Can you work these out from the model? Positions are in its coordinate system, mm. A direction names the side the tool comes from. Round coordinates to 2 decimals unless told otherwise and drop trailing zeros. Order: outer loops, then holes, each group sorted by start corner. A loop starts at its lowest first (then second) coordinate and runs counter-clockwise, first axis right, second up. Notation, with made-up numbers: (24, 29) - (75, 29) arc R22 cw to (75, 46) - close; hole circle Ø3 at (59.5, -22). An arc over 180 degrees is marked (long way). Write item = value, one per line.
from build123d import *

# Parameters (mm, degrees)
SKETCH1_R            = 3.5
BOSS_EXTRUDE1_DEPTH  = 5
SKETCH12_R           = 8.25
SKETCH12_R_2         = 3.5
BOSS_EXTRUDE6_DEPTH  = 5
BOSS_EXTRUDE9_DEPTH  = 5
CIRPATTERN2_COUNT    = 10
CUT_EXTRUDE1_START   = -10
SKETCH14_R           = 3.5
CUT_EXTRUDE1_DEPTH   = 10
SKETCH17_R           = 8.25
SKETCH17_R_2         = 3.5
BOSS_EXTRUDE10_DEPTH = 18


with BuildPart() as part:
    # Sketch1 → Boss-Extrude1 (new body)
    with BuildSketch(Plane(origin=(0, 0, 0), x_dir=(1, 0, 0), z_dir=(0, 1, 0))):
        with Locations(Location((0, 0, 0), (0, 0, 270))):
            Circle(SKETCH1_R)
    extrude(amount=BOSS_EXTRUDE1_DEPTH)

    # Sketch14 → Cut-Extrude1 (cut)
    with BuildSketch(Plane(origin=(0, 5, 0), x_dir=(1, 0, 0), z_dir=(0, 1, 0)).offset(CUT_EXTRUDE1_START)):
        with Locations(Location((0, 0, 0), (0, 0, 90))):
            Circle(SKETCH14_R)
    extrude(amount=CUT_EXTRUDE1_DEPTH, mode=Mode.SUBTRACT)


with BuildPart() as body_2:
    # Sketch12 → Boss-Extrude6 (new body)
    with BuildSketch(Plane(origin=(0, 5, 0), x_dir=(-1, 0, 0), z_dir=(0, -1, 0))):
        with Locations(Location((0, 0, 0), (0, 0, 90))):
            Circle(SKETCH12_R)
        with Locations(Location((0, 0, 0), (0, 0, 90))):
            Circle(SKETCH12_R_2, mode=Mode.SUBTRACT)
    extrude(amount=BOSS_EXTRUDE6_DEPTH)



with BuildPart() as body_3:
    # Sketch13 → Boss-Extrude9 (new body)
    with BuildSketch(Plane.XZ):
        with BuildLine():
            Line((1.7, 8.072948656), (0.86, 10.213858233))
            Line((0.86, 10.213858233), (-0.86, 10.213858233))
            Line((-0.86, 10.213858233), (-1.7, 8.072948656))
            ThreePointArc((-1.7, 8.072948656), (0, 8.25), (1.7, 8.072948656))
        make_face()
    extrude(amount=-BOSS_EXTRUDE9_DEPTH)


with BuildPart() as cirpattern2_1:
    # CirPattern2: pattern copy
    add(body_3.part.rotate(Axis((0, 0, 0), (0, 1, 0)), 1 * 360 / CIRPATTERN2_COUNT))


with BuildPart() as cirpattern2_2:
    # CirPattern2: pattern copy
    add(body_3.part.rotate(Axis((0, 0, 0), (0, 1, 0)), 2 * 360 / CIRPATTERN2_COUNT))


with BuildPart() as cirpattern2_3:
    # CirPattern2: pattern copy
    add(body_3.part.rotate(Axis((0, 0, 0), (0, 1, 0)), 3 * 360 / CIRPATTERN2_COUNT))


with BuildPart() as cirpattern2_4:
    # CirPattern2: pattern copy
    add(body_3.part.rotate(Axis((0, 0, 0), (0, 1, 0)), 4 * 360 / CIRPATTERN2_COUNT))


with BuildPart() as cirpattern2_5:
    # CirPattern2: pattern copy
    add(body_3.part.rotate(Axis((0, 0, 0), (0, 1, 0)), 5 * 360 / CIRPATTERN2_COUNT))


with BuildPart() as cirpattern2_6:
    # CirPattern2: pattern copy
    add(body_3.part.rotate(Axis((0, 0, 0), (0, 1, 0)), 6 * 360 / CIRPATTERN2_COUNT))


with BuildPart() as cirpattern2_7:
    # CirPattern2: pattern copy
    add(body_3.part.rotate(Axis((0, 0, 0), (0, 1, 0)), 7 * 360 / CIRPATTERN2_COUNT))


with BuildPart() as cirpattern2_8:
    # CirPattern2: pattern copy
    add(body_3.part.rotate(Axis((0, 0, 0), (0, 1, 0)), 8 * 360 / CIRPATTERN2_COUNT))


with BuildPart() as cirpattern2_9:
    # CirPattern2: pattern copy
    add(body_3.part.rotate(Axis((0, 0, 0), (0, 1, 0)), 9 * 360 / CIRPATTERN2_COUNT))


with BuildPart() as body_2_1:
    add(body_2.part)

    add(body_3.part)  # Boss-Extrude10 merges body 3

    add(cirpattern2_1.part)  # Boss-Extrude10 merges CirPattern2_1

    add(cirpattern2_2.part)  # Boss-Extrude10 merges CirPattern2_2

    add(cirpattern2_3.part)  # Boss-Extrude10 merges CirPattern2_3

    add(cirpattern2_4.part)  # Boss-Extrude10 merges CirPattern2_4

    add(cirpattern2_5.part)  # Boss-Extrude10 merges CirPattern2_5

    add(cirpattern2_6.part)  # Boss-Extrude10 merges CirPattern2_6

    add(cirpattern2_7.part)  # Boss-Extrude10 merges CirPattern2_7

    add(cirpattern2_8.part)  # Boss-Extrude10 merges CirPattern2_8

    add(cirpattern2_9.part)  # Boss-Extrude10 merges CirPattern2_9
    # Sketch17 → Boss-Extrude10 (add)
    # profile 1 of 11: a face of its own
    with BuildSketch(Plane.XZ):
        Circle(SKETCH17_R)
        with Locations(Location((0, 0, 0), (0, 0, 270))):
            Circle(SKETCH17_R_2, mode=Mode.SUBTRACT)
    # profile 2 of 11: a face of its own
    with BuildSketch(Plane.XZ):
        with BuildLine():
            ThreePointArc((-1.7, 8.072948656), (0, 8.25), (1.7, 8.072948656))
            Line((1.7, 8.072948656), (0.86, 10.213858233))
            Line((0.86, 10.213858233), (-0.86, 10.213858233))
            Line((-0.86, 10.213858233), (-1.7, 8.072948656))
        make_face()
    # profile 3 of 11: a face of its own
    with BuildSketch(Plane.XZ):
        with BuildLine():
            ThreePointArc((-6.120489053, 5.531917728), (-4.849228331, 6.674390204), (-3.369831272, 7.530387586))
            Line((-3.369831272, 7.530387586), (-5.307800623, 8.768680205))
            Line((-5.307800623, 8.768680205), (-6.699309853, 7.757689572))
            Line((-6.699309853, 7.757689572), (-6.120489053, 5.531917728))
        make_face()
    # profile 4 of 11: a face of its own
    with BuildSketch(Plane.XZ):
        with BuildLine():
            Line((-9.979711044, 2.338347168), (-8.203159315, 0.877882252))
            ThreePointArc((-8.203159315, 0.877882252), (-7.846216259, 2.549390204), (-7.152501534, 4.111474407))
            Line((-7.152501534, 4.111474407), (-9.448201814, 3.974164376))
            Line((-9.448201814, 3.974164376), (-9.979711044, 2.338347168))
        make_face()
    # profile 5 of 11: a face of its own
    with BuildSketch(Plane.XZ):
        with BuildLine():
            Line((-9.448201814, -3.974164376), (-7.152501534, -4.111474407))
            ThreePointArc((-7.152501534, -4.111474407), (-7.846216259, -2.549390204), (-8.203159315, -0.877882252))
            Line((-8.203159315, -0.877882252), (-9.979711044, -2.338347168))
            Line((-9.979711044, -2.338347168), (-9.448201814, -3.974164376))
        make_face()
    # profile 6 of 11: a face of its own
    with BuildSketch(Plane.XZ):
        with BuildLine():
            Line((-5.307800623, -8.768680205), (-3.369831272, -7.530387586))
            ThreePointArc((-3.369831272, -7.530387586), (-4.849228331, -6.674390204), (-6.120489053, -5.531917728))
            Line((-6.120489053, -5.531917728), (-6.699309853, -7.757689572))
            Line((-6.699309853, -7.757689572), (-5.307800623, -8.768680205))
        make_face()
    # profile 7 of 11: a face of its own
    with BuildSketch(Plane.XZ):
        with BuildLine():
            Line((0.86, -10.213858233), (1.7, -8.072948656))
            ThreePointArc((1.7, -8.072948656), (0, -8.25), (-1.7, -8.072948656))
            Line((-1.7, -8.072948656), (-0.86, -10.213858233))
            Line((-0.86, -10.213858233), (0.86, -10.213858233))
        make_face()
    # profile 8 of 11: a face of its own
    with BuildSketch(Plane.XZ):
        with BuildLine():
            Line((6.699309853, -7.757689572), (6.120489053, -5.531917728))
            ThreePointArc((6.120489053, -5.531917728), (4.849228331, -6.674390204), (3.369831272, -7.530387586))
            Line((3.369831272, -7.530387586), (5.307800623, -8.768680205))
            Line((5.307800623, -8.768680205), (6.699309853, -7.757689572))
        make_face()
    # profile 9 of 11: a face of its own
    with BuildSketch(Plane.XZ):
        with BuildLine():
            Line((7.152501534, -4.111474407), (9.448201814, -3.974164376))
            Line((9.448201814, -3.974164376), (9.979711044, -2.338347168))
            Line((9.979711044, -2.338347168), (8.203159315, -0.877882252))
            ThreePointArc((8.203159315, -0.877882252), (7.846216259, -2.549390204), (7.152501534, -4.111474407))
        make_face()
    # profile 10 of 11: a face of its own
    with BuildSketch(Plane.XZ):
        with BuildLine():
            ThreePointArc((7.152501534, 4.111474407), (7.846216259, 2.549390204), (8.203159315, 0.877882252))
            Line((8.203159315, 0.877882252), (9.979711044, 2.338347168))
            Line((9.979711044, 2.338347168), (9.448201814, 3.974164376))
            Line((9.448201814, 3.974164376), (7.152501534, 4.111474407))
        make_face()
    # profile 11 of 11: a face of its own
    with BuildSketch(Plane.XZ):
        with BuildLine():
            ThreePointArc((3.369831272, 7.530387586), (4.849228331, 6.674390204), (6.120489053, 5.531917728))
            Line((6.120489053, 5.531917728), (6.699309853, 7.757689572))
            Line((6.699309853, 7.757689572), (5.307800623, 8.768680205))
            Line((5.307800623, 8.768680205), (3.369831272, 7.530387586))
        make_face()
    extrude(amount=BOSS_EXTRUDE10_DEPTH)


solid = body_2_1.part
(1) If we section it at A-A (x = 0): Write out the boundary of the cut face in (y, z).
Computed:
outline = (-18, -10.21) - (5, -10.21) - (5, -3.5) - (-18, -3.5) - close; (-18, 3.5) - (5, 3.5) - (5, 10.21) - (-18, 10.21) - close
(2) Thinking about a two-plate mould opening in Z: for faces 1 (the face through (8.25, -6.34, -0.01)), 2 (the face through (0, -7, -10.214)), 3 (the face through (2.561, -6.339, 7.842)), which applies, +Z half, -Z half, draft (parallel to the pull), parting line (faces both ways), or undercut?
Computed:
face_1 = undercut
face_2 = -Z half
face_3 = +Z half
(3) On a 3-axis mill with a long thin cutter (end or side, diameter ignored), from which of +Z, -Z, +X, -X, +Y, -Y can I reach the whole of each face in a straight line? I mean faces 4 (the face through (-3.417, -6.339, 0.759)), 5 (the face through (-2.561, -6.339, -7.842)), 6 (the face through (-1.274, -6.661, 9.158)). Say none if no direction works.
Computed:
face_4 = +Y, -Y
face_5 = -Z, +Y, -Y
face_6 = +Z, +Y, -Y
(4) Will these pins go through, and if not, where does the flat tip stop? P1, Ø8, axis at x = 0, z = 0, coming from the -Y side; P2, Ø3, axis at y = -10, z = 5, coming from the +X side; P3, Ø1.5, axis at x = 4, y = -12.5, coming from the +Z side.
Computed:
P1 = -18
P2 = 9.6
P3 = 8.41
(5) If I drill on line 1 (X direction, y = -11, z = 8.5); line 2 (X direction, y = -7, z = -0.5); line 3 (X direction, y = -4.25, z = -1.25), over which ranges is the centre line in solid material (lowest first)? Write a range as from..to.
Computed:
line_1 = -5.68..-4.89, -1.53..1.53, 4.89..5.68
line_2 = -8.23..-3.46, 3.46..8.23
line_3 = -8.66..-3.27, 3.27..8.66
(6) If we section it at B-B (z = 0): Write out the boundary of the cut face in (x, y), plus the area to 4 significant figures.
Computed:
outline = (-8.25, -18) - (-3.5, -18) - (-3.5, 5) - (-8.25, 5) - close; (3.5, -18) - (8.25, -18) - (8.25, 5) - (3.5, 5) - close
area = 218.5 mm^2
